```python
from build123d import *

# Parameters (mm, degrees)
F1_DEPTH = 90
F2_R     = 13
F2_R_2   = 7.687325
F2_R_3   = 6.979282
F3_DEPTH = 26.8


with BuildPart() as f1:
    # F0 (on Right) → F1 (new body)
    with BuildSketch(Plane.YZ):
        Polygon((-43.438557, -7.128176), (-43.438557, -9.628176), (34.561443, -9.628176), (34.561443, -7.128176), (40.561443, -7.128176), (40.561443, 17.171824), (-49.438557, 17.171824), (-49.438557, -7.128176), align=None)
    extrude(amount=F1_DEPTH)

    # F2 (on face) → F3 (cut, through all)
    with BuildSketch(Plane.XY.offset(17.171824)):
        with Locations((75, 25.561443)):
            Circle(F2_R)
        with Locations((15, -34.438557)):
            Circle(F2_R)
        with Locations((75, -34.438557)):
            Circle(F2_R)
        with Locations((45, -34.438557)):
            Circle(F2_R_2)
        with Locations((45, 25.561443)):
            Circle(F2_R_3)
        with Locations((15, 25.561443)):
            Circle(F2_R)
    extrude(amount=-F3_DEPTH, mode=Mode.SUBTRACT)


solid = f1.part
```
Here's how the part is built. I have some questions about the finished solid (model axes, mm). A direction names the side the tool comes from. Coordinates: 2 decimals unless noted, no trailing zeros. Write each loop counter-clockwise with the first axis right and the second up, starting at its lowest first coordinate (ties: lowest second). Pieces come first, ordered by that corner, then holes. Notation, with made-up numbers: (35, 72) - (54, 72) arc R10 ccw to (54, 90) - close; hole circle Ø6 at (-13.5, -6.75). An arc over 180 degrees is marked (long way). One line per item, written item: value.
1) On a 3-axis mill with a long thin cutter (end or side, diameter ignored), from which of +Z, -Z, +X, -X, +Y, -Y can I reach the whole of each face in a straight line? I mean faces 1 (the flat face through (3, 34.561, -8)), 2 (the cylindrical face through (38.9, -39.116, 3.959)), 3 (the flat face through (44, -46, -7.128)). Say none if no direction works.
Model answer:
face 1: -Z, +X, -X, +Y
face 2: +Z, -Z
face 3: -Z, +X, -X, -Y
2) Suppose I cut it at A-A on x = 15. Write out the boundary of the cut face in (y, z).
Model answer:
outline: (-49.44, -7.13) - (-47.44, -7.13) - (-47.44, 17.17) - (-49.44, 17.17) - close; (-21.44, -9.63) - (12.56, -9.63) - (12.56, 17.17) - (-21.44, 17.17) - close; (38.56, -7.13) - (40.56, -7.13) - (40.56, 17.17) - (38.56, 17.17) - close
3) Suppose I cut it at D-D on x = 45. Write out the boundary of the cut face in (y, z), and give its area (3 significant figures).
Model answer:
outline: (-49.44, -7.13) - (-43.44, -7.13) - (-43.44, -9.63) - (-42.13, -9.63) - (-42.13, 17.17) - (-49.44, 17.17) - close; (-26.75, -9.63) - (18.58, -9.63) - (18.58, 17.17) - (-26.75, 17.17) - close; (32.54, -9.63) - (34.56, -9.63) - (34.56, -7.13) - (40.56, -7.13) - (40.56, 17.17) - (32.54, 17.17) - close
area: 1,600 mm²
4) Suppose I cut it at C-C on z = 1.5. Write out the boundary of the cut face in (x, y), and give its area (3 significant figures).
Model answer:
outline: (0, -49.44) - (90, -49.44) - (90, 40.56) - (0, 40.56) - close; hole circle Ø26 at (15, -34.44); hole circle Ø26 at (15, 25.56); hole circle Ø15.37 at (45, -34.44); hole circle Ø13.96 at (45, 25.56); hole circle Ø26 at (75, -34.44); hole circle Ø26 at (75, 25.56)
area: 5,640 mm²
5) I'm going to push flat-ended pins straight in: P1, Ø1.2, axis at x = 88.5, z = -8, coming from the -Y side; P2, Ø1.2, axis at x = 41, z = -9, coming from the +Y side. Where does each tip first touch, or does it pass through?
Model answer:
P1: stops at y = -43.44
P2: stops at y = 34.56
6) I need wall thicknesses on line 1 along Y through (x, z) = (75, 14); line 2 along X through (y, z) = (-24, 14); line 3 along X through (y, z) = (32, 0.5). Which ranges of each line are inside material? Lowest first, please.
Model answer:
line 1: y = -49.44 to -47.44, -21.44 to 12.56, 38.56 to 40.56
line 2: x = 0 to 7.25, 22.75 to 67.25, 82.75 to 90
line 3: x = 0 to 3.71, 26.29 to 42.31, 47.69 to 63.71, 86.29 to 90
7) Suppose I cut it at B-B on y = -35.5. Write out the boundary of the cut face in (x, z).
Model answer:
outline: (0, -9.63) - (2.04, -9.63) - (2.04, 17.17) - (0, 17.17) - close; (27.96, -9.63) - (37.39, -9.63) - (37.39, 17.17) - (27.96, 17.17) - close; (52.61, -9.63) - (62.04, -9.63) - (62.04, 17.17) - (52.61, 17.17) - close; (87.96, -9.63) - (90, -9.63) - (90, 17.17) - (87.96, 17.17) - close
8) We'd pull the mould along Y, two halves only. Please class faces 4 (the cylindrical face through (72.18, 12.87, 3.96)), 5 (the cylindrical face through (44.09, 32.48, 3.96)), 6 (the flat face through (44, -49.439, 5)), 7 (the flat face through (44, -5, -9.628)): pulls with the +Y half, pulls with the -Y half, needs draft (parallel to the pull), parting line crosses it, or undercut.
Model answer:
face 4: undercut
face 5: undercut
face 6: pulls with the -Y half
face 7: needs draft
